from build123d import *

# Parameters (mm, degrees)
BASE_FLANGE1_START = -94.375
BASE_FLANGE1_DEPTH = 188.75
CUT_EXTRUDE1_REACH = 246.612


# Read off the part's stored shape, not the designer's step: Base-Flange1
with BuildPart() as part:
    # Base-Flange1 outline → Base-Flange1 (new body)
    with BuildSketch(Plane.XY.offset(BASE_FLANGE1_START)):
        with BuildLine():
            Line((-332.415300569, 2.8956), (-360.542189104, 51.6128))
            Line((-360.542189104, 51.6128), (-361.95, 50.8))
            Line((-361.95, 50.8), (-333.823111466, 2.0828))
            ThreePointArc((-333.823111466, 2.0828), (-332.298396044, 0.558084578), (-330.215596044, 0))
            Line((-330.215596044, 0), (-144.5156, 0))
            ThreePointArc((-144.5156, 0), (-141.570075992, 1.220075992), (-140.35, 4.1656))
            Line((-140.35, 4.1656), (-140.35, 46.6344))
            ThreePointArc((-140.35, 46.6344), (-141.570075992, 49.579924008), (-144.5156, 50.8))
            Line((-144.5156, 50.8), (-165.35, 50.8))
            Line((-165.35, 50.8), (-165.35, 49.1744))
            Line((-165.35, 49.1744), (-144.5156, 49.1744))
            ThreePointArc((-144.5156, 49.1744), (-142.719548776, 48.430451224), (-141.9756, 46.6344))
            Line((-141.9756, 46.6344), (-141.9756, 4.1656))
            ThreePointArc((-141.9756, 4.1656), (-142.719548776, 2.369548776), (-144.5156, 1.6256))
            Line((-144.5156, 1.6256), (-330.215596044, 1.6256))
            ThreePointArc((-330.215596044, 1.6256), (-331.485596044, 1.965895474), (-332.415300569, 2.8956))
        make_face()
    extrude(amount=BASE_FLANGE1_DEPTH)

    # Sketch15 → Cut-Extrude1 (cut, up to next)
    with BuildSketch(Plane(origin=(-249.465454744, -144.02894745, 0), x_dir=(0, 0, 1), z_dir=(-0.8660254037844362, -0.5000000000000044, 0)), mode=Mode.PRIVATE) as cut_extrude1_sk1:
        with BuildLine():
            Line((66.825, 172.969090512), (66.825, 177.969090512))
            ThreePointArc((66.825, 177.969090512), (70, 181.144090512), (73.175, 177.969090512))
            Line((73.175, 177.969090512), (73.175, 172.969090512))
            ThreePointArc((73.175, 172.969090512), (70, 169.794090512), (66.825, 172.969090512))
        make_face()
    cut_extrude1_tool1 = extrude(cut_extrude1_sk1.sketch, amount=-CUT_EXTRUDE1_REACH, mode=Mode.PRIVATE) & part.part
    # Sketch15 → Cut-Extrude1 (cut, up to next)
    with BuildSketch(Plane(origin=(-249.465454744, -144.02894745, 0), x_dir=(0, 0, 1), z_dir=(-0.8660254037844362, -0.5000000000000044, 0)), mode=Mode.PRIVATE) as cut_extrude1_sk2:
        with BuildLine():
            Line((-66.825, 172.969090512), (-66.825, 177.969090512))
            ThreePointArc((-66.825, 177.969090512), (-70, 181.144090512), (-73.175, 177.969090512))
            Line((-73.175, 177.969090512), (-73.175, 172.969090512))
            ThreePointArc((-73.175, 172.969090512), (-70, 169.794090512), (-66.825, 172.969090512))
        make_face()
    cut_extrude1_tool2 = extrude(cut_extrude1_sk2.sketch, amount=-CUT_EXTRUDE1_REACH, mode=Mode.PRIVATE) & part.part
    add(cut_extrude1_tool1.solids().sort_by_distance((-337.2, 7.931743, 70))[0], mode=Mode.SUBTRACT)
    add(cut_extrude1_tool2.solids().sort_by_distance((-337.2, 7.931743, -70))[0], mode=Mode.SUBTRACT)


solid = part.part
The model under review builds one solid part; all positions refer to its coordinate system, in mm. A direction names the side the tool comes from. Round coordinates to 2 decimals unless told otherwise and drop trailing zeros. Loops run counter-clockwise (first coordinate to the right, second up) from the corner with the lowest first, then second, coordinate; pieces in that order, holes last. Notation, with made-up numbers: M 30.5,7.5 L 70.5,7.5 A31 cw 70.5,32.5 Z; hole C 2,83.25 d10. An arc over 180 degrees is marked long. Answer as CSV lines item,"result".
1. For faces 5 (the face through (-140.35, 25, -1)), 6 (the face through (-141.976, 26, -1)), 7 (the face through (-155, 50.8, -1)), list the 3-axis set-ups (+Z, -Z, +X, -X, +Y, -Y) from which the entire face can be reached by the end or side of a thin tool; tool diameter is ignored.
Outcome:
face 5,"+Z, -Z, +X, +Y, -Y"
face 6,"+Z, -Z"
face 7,"+Z, -Z, +X, +Y"
2. We need section C-C (x = -242). Give the boundary of the cut face in (y, z) (3 decimals).
Outcome:
outline,"M 0,-94.375 L 1.626,-94.375 L 1.626,94.375 L 0,94.375 Z"
3. Insertion check: pin 1 Ø16.5 at (x, z) = (-153.5, -33.5) entering from +Y; pin 2 Ø0.8 at (y, z) = (50, 28) entering from -X; pin 3 Ø12.5 at (y, z) = (18, -37) entering from -X. Each pin has a flat end and moves straight along its axis. Give the tip position at first contact, or say it passes through.
Outcome:
pin 1,"stops at y = 50.8"
pin 2,"stops at x = -361.72"
pin 3,"stops at x = -346.62"
4. We need section B-B (z = 82.5). Give the boundary of the cut face in (x, y), plus the area to 3 significant figures.
Outcome:
outline,"M -361.95,50.8 L -333.82,2.08 A4.17 ccw -330.22,0 L -144.52,0 A4.17 ccw -140.35,4.17 L -140.35,46.63 A4.17 ccw -144.52,50.8 L -165.35,50.8 L -165.35,49.17 L -144.52,49.17 A2.54 cw -141.98,46.63 L -141.98,4.17 A2.54 cw -144.52,1.63 L -330.22,1.63 A2.54 cw -332.42,2.9 L -360.54,51.61 Z"
area,"519 mm2"
5. To check wall thickness, follow L1, parallel to Y at x = -182, z = 24; L2, parallel to X at y = 24.5, z = -26; L3, parallel to X at y = 18.5, z = -30.5. State the ranges of each line that lie inside material, in increasing order. Write a range as [from, to].
Outcome:
L1,"y = [0, 1.63]"
L2,"x = [-346.77, -344.89], [-141.98, -140.35]"
L3,"x = [-343.3, -341.42], [-141.98, -140.35]"
6. Draft analysis for pull direction X (two halves, no side actions). For faces 1 (the face through (-348.08, 26.78, -1.32)), 2 (the face through (-346.28, 26.91, -1.32)), 3 (the face through (-252, 1, -94.375)), 4 (the face through (-155, 49.174, -1)), state which applies: pulls with the +X half, pulls with the -X half, needs draft (parallel to the pull), parting line crosses it, or undercut.
Outcome:
face 1,"pulls with the -X half"
face 2,"undercut"
face 3,"needs draft"
face 4,"undercut"
7. We need section A-A (y = 22). Give the boundary of the cut face in (x, z) (3 decimals), plus the area to 3 significant figures.
Outcome:
outline,"M -345.322,-94.375 L -343.445,-94.375 L -343.445,94.375 L -345.322,94.375 Z; M -141.976,-94.375 L -140.35,-94.375 L -140.35,94.375 L -141.976,94.375 Z"
area,"661 mm2"
